```python
from build123d import *

# Parameters (mm, degrees)
BOSS_EXTRUDE1_DEPTH       = 100
CUT_EXTRUDE8_DEPTH        = 100
CUT_EXTRUDE8_DEPTH_BACK   = 100
SKETCH4_W                 = 25
SKETCH4_H                 = 55
CUT_EXTRUDE9_DEPTH        = 10
CUT_EXTRUDE10_DEPTH       = 10
SKETCH7_W                 = 80
SKETCH7_H                 = 65
BOSS_EXTRUDE2_DEPTH       = 10
SKETCH8_W                 = 100
SKETCH8_H                 = 20
CUT_EXTRUDE11_DEPTH       = 10
BOSS_EXTRUDE11_DEPTH      = 90
BOSS_EXTRUDE11_DEPTH_BACK = 10
SKETCH9_W                 = 25
SKETCH9_H                 = 15
CUT_EXTRUDE16_DEPTH       = 12.5
CUT_EXTRUDE16_DEPTH_BACK  = 12.5
SKETCH10_OUTSIDE_W        = 131.682
SKETCH10_OUTSIDE_H        = 131.682


with BuildPart() as part:
    # Sketch2 → Boss-Extrude1 (new body)
    with BuildSketch(Plane(origin=(0, 0, 0), x_dir=(1, 0, 0), z_dir=(0, 1, 0))):
        Polygon((-40, 22.5), (-40, -12.5), (40, -12.5), (40, 22.5), (50, 22.5), (50, -22.5), (-50, -22.5), (-50, 22.5), align=None)
    extrude(amount=BOSS_EXTRUDE1_DEPTH)

    # Sketch4 → Cut-Extrude8 (cut, two sides: drawn at the far end of the back side and taken through both)
    with BuildSketch(Plane(origin=(0, 0, 0), x_dir=(0, 0, -1), z_dir=(1, 0, 0)).offset(-CUT_EXTRUDE8_DEPTH_BACK)):
        with Locations((0, 27.5)):
            Rectangle(SKETCH4_W, SKETCH4_H)
    extrude(amount=CUT_EXTRUDE8_DEPTH + CUT_EXTRUDE8_DEPTH_BACK, mode=Mode.SUBTRACT)

    # Sketch5 → Cut-Extrude9 (cut)
    with BuildSketch(Plane.XY.offset(22.5)):
        Polygon((-50, 50), (0, 0), (-50, 0), align=None)
    extrude(amount=-CUT_EXTRUDE9_DEPTH, mode=Mode.SUBTRACT)

    # Sketch6 → Cut-Extrude10 (cut)
    with BuildSketch(Plane.XY.offset(22.5)):
        Polygon((0, 0), (50, 50), (50, 0), align=None)
    extrude(amount=-CUT_EXTRUDE10_DEPTH, mode=Mode.SUBTRACT)


with BuildPart() as body_2:
    # Sketch7 → Boss-Extrude2 (new body)
    with BuildSketch(Plane(origin=(0, 0, -22.5), x_dir=(-1, 0, 0), z_dir=(0, 0, -1))):
        with Locations((0, 32.5)):
            Rectangle(SKETCH7_W, SKETCH7_H)
    extrude(amount=-BOSS_EXTRUDE2_DEPTH)


with BuildPart() as cut_extrude11_tool:
    # Sketch8 → Cut-Extrude11 (new body)
    with BuildSketch(Plane(origin=(0, 0, -22.5), x_dir=(-1, 0, 0), z_dir=(0, 0, -1))):
        with Locations((0, 10)):
            Rectangle(SKETCH8_W, SKETCH8_H)
    extrude(amount=-CUT_EXTRUDE11_DEPTH)


with BuildPart() as part_1:
    add(part.part)

    # Cut-Extrude11: cut by cut_extrude11_tool
    add(cut_extrude11_tool.part, mode=Mode.SUBTRACT)



with BuildPart() as body_2_1:
    add(body_2.part)

    # Cut-Extrude11: cut by cut_extrude11_tool
    add(cut_extrude11_tool.part, mode=Mode.SUBTRACT)


with BuildPart() as part_2:
    add(part_1.part)

    add(body_2_1.part)  # Boss-Extrude11 merges body 2
    # Sketch9 → Boss-Extrude11 (add, two sides: drawn at the far end of the back side and taken through both)
    with BuildSketch(Plane(origin=(-40, 0, 0), x_dir=(0, 0, -1), z_dir=(1, 0, 0)).offset(-BOSS_EXTRUDE11_DEPTH_BACK)):
        with Locations((0, 57.5)):
            Rectangle(SKETCH9_W, SKETCH9_H)
    extrude(amount=BOSS_EXTRUDE11_DEPTH + BOSS_EXTRUDE11_DEPTH_BACK)

    # Sketch10 outside → Cut-Extrude16 (cut, two sides: drawn at the far end of the back side and taken through both)
    with BuildSketch(Plane.XY.offset(-CUT_EXTRUDE16_DEPTH_BACK)):
        with Locations((0, 50)):
            Rectangle(SKETCH10_OUTSIDE_W, SKETCH10_OUTSIDE_H)
        with BuildLine():
            Line((50, 55), (46.160254038, 55))
            ThreePointArc((46.160254038, 55), (37.5, 50), (28.839745962, 55))
            Line((28.839745962, 55), (-28.839745962, 55))
            ThreePointArc((-28.839745962, 55), (-37.5, 50), (-46.160254038, 55))
            Line((-46.160254038, 55), (-50, 55))
            Line((-50, 55), (-50, 100))
            Line((-50, 100), (-40, 100))
            Line((-40, 100), (-40, 65))
            Line((-40, 65), (40, 65))
            Line((40, 65), (40, 100))
            Line((40, 100), (50, 100))
            Line((50, 100), (50, 55))
        make_face(mode=Mode.SUBTRACT)
    extrude(amount=CUT_EXTRUDE16_DEPTH + CUT_EXTRUDE16_DEPTH_BACK, mode=Mode.SUBTRACT)


solid = part_2.part
```
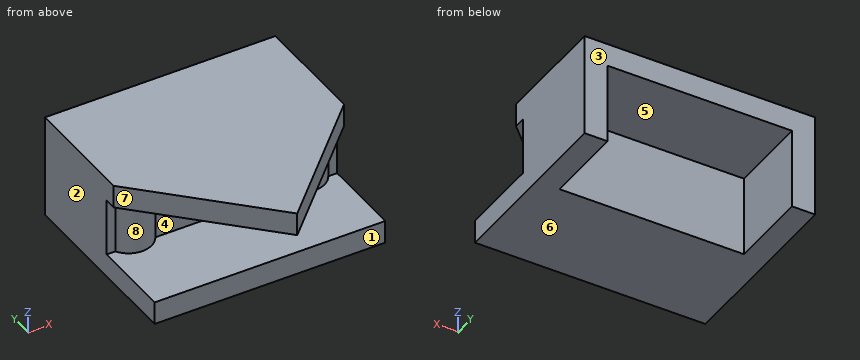
Check sheet for the modelled part. Datum: model origin and axes. Units: mm. Face numbers are marked on the shaded views. A direction names the side the tool comes from. Round coordinates to 2 decimals unless told otherwise and drop trailing zeros. Write each loop counter-clockwise with the first axis right and the second up, starting at its lowest first coordinate (ties: lowest second). Pieces come first, ordered by that corner, then holes. Notation, with made-up numbers: (-28, -40) -> (-14, -40) arc R23 ccw to (-14, -32) -> close; hole circle Ø11 at (37, 46.5). An arc over 180 degrees is marked (long way). One line per question, with ' | ' between items. Start each with the question number.
1. Depth check by flat-ended pin: pin 1 (1.9 mm diameter, centred on x = 49, z = 1, fed in from -Y); pin 2 (6 mm diameter, centred on y = 29, z = 17.5, fed in from +X); pin 3 (17.5 mm diameter, centred on x = -9, z = -4.5, fed in from +Y). Enter the tip coordinate at first touch or a pass-through.
2. Scan lines: line 1 along X through (y, z) = (76.5, -19.5); line 2 along Y through (x, z) = (-8, -13); line 3 along Z through (x, y) = (-18.5, 25). Record each from-to range of solid material in increasing order. Write a range as from..to.
3. Set-up check for the marked faces 1, 2, 3, 4 and 5: record each of +Z, -Z, +X, -X, +Y, -Y from which the full face is reachable in a straight line by a thin tool's end or side.
4. Sectioned sample at B-B, the plane x = -23.5. Record the cut outline in (y, z).
5. Sectioned sample at C-C, the plane z = -20. Record the cut outline in (x, y), then the cut area to 3 significant figures.
6. Sectioned sample at A-A, the plane y = 31. Record the cut outline in (x, z), then the cut area to 3 significant figures.
7. Sectioned sample at D-D, the plane y = 88. Record the cut outline in (x, z).
8. Release check for a two-part mould opening along Z. For the marked faces 6, 7 and 8 record: +Z half, -Z half, draft (parallel to the pull), parting line (faces both ways), or undercut.
Taken from the geometry:
1) pin 1: stops at y = 55 | pin 2: stops at x = 32 | pin 3: stops at y = 65
2) line 1: x = -50..-40, 40..50 | line 2: y = 20..65 | line 3: z = -22.5..-12.5, 12.5..22.5
3) face 1: -Z, +X, -X, -Y | face 2: +Z, -Z, -X, +Y, -Y | face 3: +Z, -Z, +X, -X, +Y | face 4: -Y | face 5: -Z, +Y
4) outline: (20, -22.5) -> (65, -22.5) -> (65, 12.5) -> (100, 12.5) -> (100, 22.5) -> (23.5, 22.5) -> (23.5, 12.5) -> (55, 12.5) -> (55, -12.5) -> (20, -12.5) -> close
5) outline: (-50, 20) -> (50, 20) -> (50, 100) -> (40, 100) -> (40, 65) -> (-40, 65) -> (-40, 100) -> (-50, 100) -> close | area: 5,200 mm^2
6) outline: (-50, -22.5) -> (50, -22.5) -> (50, -12.5) -> (-50, -12.5) -> close; (-31, 12.5) -> (31, 12.5) -> (31, 22.5) -> (-31, 22.5) -> close | area: 1,620 mm^2
7) outline: (-50, -22.5) -> (-40, -22.5) -> (-40, 12.5) -> (40, 12.5) -> (40, -22.5) -> (50, -22.5) -> (50, 22.5) -> (-50, 22.5) -> close
8) face 6: -Z half | face 7: draft | face 8: undercut
